from build123d import *

# Parameters (mm, degrees)
F1_DEPTH = 25.4
F2_R     = 4.699
F3_DEPTH = 19.05


with BuildPart() as f1:
    # F0 (on Front) → F1 (new body)
    with BuildSketch(Plane.XZ):
        Polygon((-38.1, -34.925), (38.1, -34.925), (38.1, 34.925), (14.3002, 34.925), (14.3002, 6.35), (-14.2748, 6.35), (-14.2748, 34.925), (-38.1, 34.925), align=None)
    extrude(amount=F1_DEPTH)

    # F2 (on face) → F3 (join)
    with BuildSketch(Plane(origin=(0, 0, -34.925), x_dir=(1, 0, 0), z_dir=(0, 0, -1))):
        Polygon((-38.1, 25.4), (38.1, 25.4), (38.1, 82.55), (38.1, 95.25), (25.4, 95.25), (-25.4, 95.25), (-38.1, 95.25), (-38.1, 82.55), align=None)
        with Locations((-25.4, 82.55)):
            Circle(F2_R, mode=Mode.SUBTRACT)
        with Locations((25.4, 82.55)):
            Circle(F2_R, mode=Mode.SUBTRACT)
        Polygon((38.1, -12.7), (38.1, 0), (-38.1, 0), (-38.1, -25.4), (25.4, -25.4), (38.1, -25.4), align=None)
        with Locations((-25.4, -12.7)):
            Circle(F2_R, mode=Mode.SUBTRACT)
        with Locations((25.4, -12.7)):
            Circle(F2_R, mode=Mode.SUBTRACT)
    extrude(amount=-F3_DEPTH)


solid = f1.part
Read the model definition and answer for the solid it produces. Units are mm, in the model's axes. A direction names the side the tool comes from. Coordinates: 2 decimals unless noted, no trailing zeros. Loops run counter-clockwise (first coordinate to the right, second up) from the corner with the lowest first, then second, coordinate; pieces in that order, holes last. Notation, with made-up numbers: (50, -39.5) - (100, -39.5) arc R15 ccw to (100, -22.5) - close; hole circle Ø7 at (34, 88). An arc over 180 degrees is marked (long way). Answer in a Markdown table with one row per item.
Q1. Find section D-D on z = -24. Write down the section's boundary in (x, y).
Here are the results:
| item | result |
|---|---|
| outline | (-38.1, -95.25) - (38.1, -95.25) - (38.1, 25.4) - (-38.1, 25.4) - close; hole circle Ø9.4 at (-25.4, -82.55); hole circle Ø9.4 at (-25.4, 12.7); hole circle Ø9.4 at (25.4, -82.55); hole circle Ø9.4 at (25.4, 12.7) |
Q2. Straight lines are drawn through the part: line 1 along X through (y, z) = (-82.55, -27); line 2 along Y through (x, z) = (-25, -25); line 3 along X through (y, z) = (12, -28). For each, find the intervals that lie inside material, in ascending order. Write a range as [from, to].
Here are the results:
| item | result |
|---|---|
| line 1 | x = [-38.1, -30.1], [-20.7, 20.7], [30.1, 38.1] |
| line 2 | y = [-95.25, -87.23], [-77.87, 8.02], [17.38, 25.4] |
| line 3 | x = [-38.1, -30.05], [-20.75, 20.75], [30.05, 38.1] |
Q3. Given P1, Ø15, axis at x = -25.4, y = -82.55, coming from the +Z side (3 decimals); P2, Ø7.5, axis at x = 5, y = -14, coming from the +Z side; P3, Ø4, axis at x = 25.5, z = 12, coming from the -Y side, each flat-ended and moving along its own axis, determine where each tip first touches the part or whether it passes through.
Here are the results:
| item | result |
|---|---|
| P1 | stops at z = -15.875 |
| P2 | stops at z = 6.35 |
| P3 | stops at y = -25.4 |
Q4. The mould has two halves that part along Y. Classify faces 1 (the flat face through (-1, 25.4, -26)), 2 (the cylindrical face through (29.882, 11.289, -25.533)), 3 (the flat face through (-38.1, -22, -16)): pulls with the +Y half, pulls with the -Y half, needs draft (parallel to the pull), parting line crosses it, or undercut.
Here are the results:
| item | result |
|---|---|
| face 1 | pulls with the +Y half |
| face 2 | undercut |
| face 3 | needs draft |
Q5. For faces 4 (the flat face through (-26, -13, 34.925)), 5 (the flat face through (14.3, -13, 21)), 6 (the flat face through (-1, 0, 4)), 7 (the cylindrical face through (-20.918, 11.289, -25.533)), 8 (the flat face through (-1, -25.4, 4)), determine the directions among +Z, -Z, +X, -X, +Y, -Y from which every point of the face is accessible in a straight line to the end or side of a thin tool.
Here are the results:
| item | result |
|---|---|
| face 4 | +Z, +X, -X, +Y, -Y |
| face 5 | +Z, +Y, -Y |
| face 6 | +Z, +X, -X, +Y |
| face 7 | +Z, -Z |
| face 8 | +Z, +X, -X, -Y |
Q6. Find section B-B on z = 21.5. Write down the section's boundary in (x, y), plus the area to 3 significant figures.
Here are the results:
| item | result |
|---|---|
| outline | (-38.1, -25.4) - (-14.27, -25.4) - (-14.27, 0) - (-38.1, 0) - close; (14.3, -25.4) - (38.1, -25.4) - (38.1, 0) - (14.3, 0) - close |
| area | 1,210 mm^2 |
Q7. Find section A-A on x = -25.4. Write down the section's boundary in (y, z) (3 decimals).
Here are the results:
| item | result |
|---|---|
| outline | (-95.25, -34.925) - (-87.249, -34.925) - (-87.249, -15.875) - (-95.25, -15.875) - close; (-77.851, -34.925) - (8.001, -34.925) - (8.001, -15.875) - (0, -15.875) - (0, 34.925) - (-25.4, 34.925) - (-25.4, -15.875) - (-77.851, -15.875) - close; (17.399, -34.925) - (25.4, -34.925) - (25.4, -15.875) - (17.399, -15.875) - close |
Q8. Find section C-C on y = 12.7. Write down the section's boundary in (x, z) (3 decimals).
Here are the results:
| item | result |
|---|---|
| outline | (-38.1, -34.925) - (-30.099, -34.925) - (-30.099, -15.875) - (-38.1, -15.875) - close; (-20.701, -34.925) - (20.701, -34.925) - (20.701, -15.875) - (-20.701, -15.875) - close; (30.099, -34.925) - (38.1, -34.925) - (38.1, -15.875) - (30.099, -15.875) - close |
